Can you work these out from the model? Positions are in its coordinate system, mm. Give positions to 0.01 mm unless a question says otherwise; leave off trailing zeros. Order: outer loops, then holes, each group sorted by start corner. A loop starts at its lowest first (then second) coordinate and runs counter-clockwise, first axis right, second up. Notation, with made-up numbers: (-34.75, -22) - (-14.75, -22) arc R19 cw to (-14.75, -4) - close; hole circle Ø8 at (22.25, -18.75). An arc over 180 degrees is marked (long way). Answer as CSV lines item,"result".
```python
from build123d import *

# Parameters (mm, degrees)
SKETCH1_W           = 266.7
SKETCH1_H           = 31.75
BOSS_EXTRUDE1_DEPTH = 31.75
SKETCH2_R           = 7.9375
CUT_EXTRUDE1_DEPTH  = 31.75
LPATTERN1_COUNT     = 9
LPATTERN1_PITCH     = 25.4
SKETCH3_R           = 2.50825
CUT_EXTRUDE2_DEPTH  = 31.75


with BuildPart() as part:
    # Sketch1 → Boss-Extrude1 (new body)
    with BuildSketch(Plane.XY):
        with Locations((-133.35, -15.875)):
            Rectangle(SKETCH1_W, SKETCH1_H)
    extrude(amount=BOSS_EXTRUDE1_DEPTH)

    # Sketch2 → Cut-Extrude1 (cut)
    with BuildSketch(Plane.XY.offset(31.75)):
        with Locations((-234.95, -15.875)):
            Circle(SKETCH2_R)
    cut_extrude1 = extrude(amount=-CUT_EXTRUDE1_DEPTH, mode=Mode.SUBTRACT)

    # LPattern1: Cut-Extrude1 ×9
    with Locations(*[(i * LPATTERN1_PITCH, 0, 0) for i in range(1, LPATTERN1_COUNT)]):
        add(cut_extrude1, mode=Mode.SUBTRACT)

    # Sketch3 → Cut-Extrude2 (cut)
    with BuildSketch(Plane.XY.offset(31.75)):
        with Locations((-260.35, -9.525)):
            Circle(SKETCH3_R)
        with Locations((-247.65, -9.525)):
            Circle(SKETCH3_R)
        with Locations((-260.35, -22.225)):
            Circle(SKETCH3_R)
        with Locations((-247.65, -22.225)):
            Circle(SKETCH3_R)
    extrude(amount=-CUT_EXTRUDE2_DEPTH, mode=Mode.SUBTRACT)


solid = part.part
```
1) I want a section at C-C on x = -61. Write out the boundary of the cut face in (y, z), plus the area to 3 significant figures.
Answer block:
outline,"(-31.75, 0) - (-22.82, 0) - (-22.82, 31.75) - (-31.75, 31.75) - close; (-8.93, 0) - (0, 0) - (0, 31.75) - (-8.93, 31.75) - close"
area,"567 mm2"
2) I want a section at A-A on x = -247.65. Write out the boundary of the cut face in (y, z).
Answer block:
outline,"(-31.75, 0) - (-24.73, 0) - (-24.73, 31.75) - (-31.75, 31.75) - close; (-19.72, 0) - (-12.03, 0) - (-12.03, 31.75) - (-19.72, 31.75) - close; (-7.02, 0) - (0, 0) - (0, 31.75) - (-7.02, 31.75) - close"
3) I'm going to push a flat-ended pin straight in: P1, Ø14.5, axis at x = -57.15, y = -15.875, coming from the +Z side. Where does the tip first touch, or does it pass through?
Answer block:
P1,"through"
4) I need wall thicknesses on line 1 along Y through (x, z) = (-57, 29); line 2 along Y through (x, z) = (-134, 8.5); line 3 along Y through (x, z) = (-260, 19). Which ranges of each line are inside material? Lowest first, please. Write a range as [from, to].
Answer block:
line 1,"[-31.75, -23.81], [-7.94, 0]"
line 2,"[-31.75, -23.79], [-7.96, 0]"
line 3,"[-31.75, -24.71], [-19.74, -12.01], [-7.04, 0]"
5) If we mould it in two halves opening along Y, with no side actions, what happens to faces 1 (the cylindrical face through (-217.48, -15.53, 16.1)), 2 (the flat face through (-135, -31.75, 16)), 3 (the flat face through (0, -16, 16))? For each: +Y half, -Y half, draft (parallel to the pull), parting line (faces both ways), or undercut.
Answer block:
face 1,"undercut"
face 2,"-Y half"
face 3,"draft"
6) I want a section at B-B on z = 7. Count the separate pieces of the cut face and the enclosed holes in it, plus the area to 3 significant figures.
Answer block:
separate pieces,"1"
enclosed holes,"13"
area,"6,610 mm2"
